from build123d import *

# Parameters (mm, degrees)
F0_W     = 1778
F0_H     = 1574.8
F1_DEPTH = 6.35
F3_DEPTH = 508
F4_W     = 12.7
F4_H     = 31.75
F5_DEPTH = 76.2
F6_R     = 6.35
F7_DEPTH = 1714.501


with BuildPart() as f1:
    # F0 (on Top) → F1 (new body)
    with BuildSketch(Plane.XY):
        Rectangle(F0_W, F0_H)
    extrude(amount=F1_DEPTH)

    # F2 (on face) → F3 (join)
    with BuildSketch(Plane.XY.offset(6.35)):
        Polygon((-889, 736.6), (-889, -787.4), (-762, -787.4), (-762, 736.6), (762, 736.6), (762, -787.4), (889, -787.4), (889, 736.6), (889, 787.4), (762, 787.4), (-762, 787.4), (-889, 787.4), align=None)
    extrude(amount=F3_DEPTH)

    # F4 (on face) → F5 (join)
    with BuildSketch(Plane.XZ.offset(787.4)):
        with Locations((-819.15, 15.875)):
            Rectangle(F4_W, F4_H)
        with Locations((819.15, 15.875)):
            Rectangle(F4_W, F4_H)
    extrude(amount=F5_DEPTH)

    # F6 (on face) → F7 (cut, through all)
    with BuildSketch(Plane(origin=(-825.5, 0, 0), x_dir=(0, -1, 0), z_dir=(-1, 0, 0))):
        with Locations((828.675, 15.875)):
            Circle(F6_R)
    extrude(amount=-F7_DEPTH, mode=Mode.SUBTRACT)


solid = f1.part
Build history of the part. All positions in model axes, mm. A direction names the side the tool comes from. Round coordinates to 2 decimals unless told otherwise and drop trailing zeros. Write each loop counter-clockwise with the first axis right and the second up, starting at its lowest first coordinate (ties: lowest second). Pieces come first, ordered by that corner, then holes. Notation, with made-up numbers: M 4.25,-10.75 L 51.25,-10.75 A26 ccw 51.25,23.25 Z; hole C -20.75,-11.5 d1. An arc over 180 degrees is marked long. Answer as a JSON object with one key per item and string values. Group by question number.
(1) Which spindle directions (+Z, -Z, +X, -X, +Y, -Y) get a long thin tool onto all of the face, cutting with end or side? Do faces 4 (the flat face through (-11, -15, 6.35)), 5 (the flat face through (-889, 11, 254)). Say none if no direction does.
(2) Cut at A-A (z = 183). Give the cut face in (x, y), and give its area (3 significant figures).
(3) Flat gauge pins, fed straight in: pin 1 (16 mm diameter, centred on y = -828, z = 18.5, fed in from +X); pin 2 (6.5 mm diameter, centred on x = 816, y = -835.5, fed in from +Z); pin 3 (14.5 mm diameter, centred on y = -828.675, z = 15.875, fed in from -X). Where does each tip first touch, or does it go through?
(4) Drill centre lines: L1, parallel to X at y = -70, z = 161; L2, parallel to Z at x = 475.5, y = 649; L3, parallel to Y at x = 650, z = 289.5. Where is each one in solid material? Low to high.
(5) Cut at C-C (x = -423). Give the cut face in (y, z).
(6) Mould opens along X. For faces 1 (the flat face through (-4, 762, 514.35)), 2 (the flat face through (889, -11, 254)), 3 (the flat face through (-11, 736.6, 257)) say: pulls with the +X half, pulls with the -X half, needs draft (parallel to the pull), parting line crosses it, or undercut.
(7) Cut at B-B (y = -459.5). Give the cut face in (x, z).
Responses:
{
 "1": {"face 4": "+Z, -Y", "face 5": "+Z, -Z, -X, +Y, -Y"},
 "2": {"outline": "M -889,-787.4 L -762,-787.4 L -762,736.6 L 762,736.6 L 762,-787.4 L 889,-787.4 L 889,787.4 L -889,787.4 Z", "area": "477,000 mm2"},
 "3": {"pin 1": "stops at x = 825.5", "pin 2": "stops at z = 31.75", "pin 3": "stops at x = -825.5"},
 "4": {"L1": "x = -889 to -762, 762 to 889", "L2": "z = 0 to 6.35", "L3": "y = 736.6 to 787.4"},
 "5": {"outline": "M -787.4,0 L 787.4,0 L 787.4,514.35 L 736.6,514.35 L 736.6,6.35 L -787.4,6.35 Z"},
 "6": {"face 1": "needs draft", "face 2": "pulls with the +X half", "face 3": "undercut"},
 "7": {"outline": "M -889,0 L 889,0 L 889,514.35 L 762,514.35 L 762,6.35 L -762,6.35 L -762,514.35 L -889,514.35 Z"}
}
